from build123d import *

# Parameters (mm, degrees)
BOSS_EXTRUDE1_DEPTH = 1
SKETCH3_R           = 3.15
BOSS_EXTRUDE2_DEPTH = 7.7
FILLET1_R           = 0.3
SKETCH4_W           = 0.65
SKETCH4_H           = 2.8
BOSS_EXTRUDE3_DEPTH = 0.3
BOSS_EXTRUDE4_DEPTH = 0.01


with BuildPart() as part:
    # Sketch2 → Boss-Extrude1 (new body)
    with BuildSketch(Plane(origin=(0, 0, 0), x_dir=(1, 0, 0), z_dir=(0, 1, 0))):
        Polygon((3.3, -3.3), (-3.3, -3.3), (-3.3, 2.25), (-2.25, 3.3), (2.25, 3.3), (3.3, 2.25), align=None)
    extrude(amount=BOSS_EXTRUDE1_DEPTH)

    # Sketch3 → Boss-Extrude2 (add)
    with BuildSketch(Plane(origin=(0, 0, 0), x_dir=(1, 0, 0), z_dir=(0, 1, 0))):
        Circle(SKETCH3_R)
    extrude(amount=BOSS_EXTRUDE2_DEPTH)

    # Fillet1
    fillet1_edges = [part.edges().sort_by_distance(p)[0] for p in [
        (-3.15, 7.7, 0),
    ]]
    fillet(fillet1_edges, radius=FILLET1_R)

    # Sketch4 → Boss-Extrude3 (add)
    with BuildSketch(Plane(origin=(0, 0, 0), x_dir=(1, 0, 0), z_dir=(0, 1, 0))):
        with Locations((0, 2.2)):
            Rectangle(SKETCH4_W, SKETCH4_H)
        with Locations((0, -2.2)):
            Rectangle(SKETCH4_W, SKETCH4_H)
    extrude(amount=BOSS_EXTRUDE3_DEPTH)

    # Sketch5 → Boss-Extrude4 (add)
    with BuildSketch(Plane(origin=(0, 7.7, 0), x_dir=(1, 0, 0), z_dir=(0, 1, 0))):
        with BuildLine():
            Line((-2.494581862, -1.378245745), (2.494581862, -1.378245745))
            ThreePointArc((2.494581862, -1.378245745), (0, -2.85), (-2.494581862, -1.378245745))
        make_face()
    extrude(amount=BOSS_EXTRUDE4_DEPTH)


solid = part.part
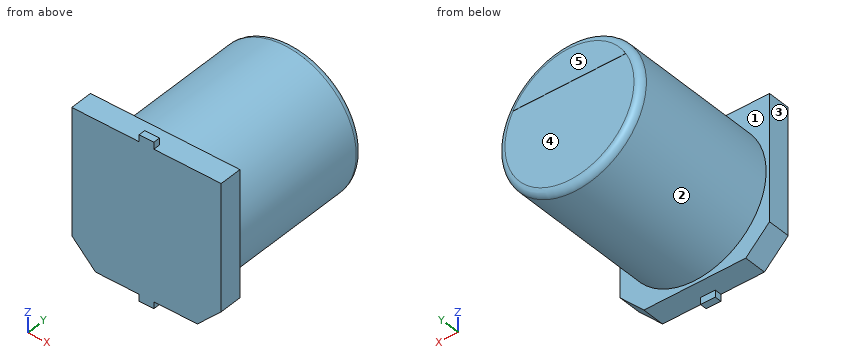
Could you check a few things on this model? Use its own coordinates, in mm. Face numbers are marked on the shaded views. A direction names the side the tool comes from. Round coordinates to 2 decimals unless told otherwise and drop trailing zeros. Write each loop counter-clockwise with the first axis right and the second up, starting at its lowest first coordinate (ties: lowest second). Pieces come first, ordered by that corner, then holes. Notation, with made-up numbers: (20.25, 24) - (33.25, 24) arc R11 ccw to (33.25, 35) - close; hole circle Ø5 at (36, 37.5). An arc over 180 degrees is marked (long way). Put each result on its own line as item: value. Start each with the question number.
(1) I want a section at B-B, the plane y = 0.5. Please give me the cut outline in (x, z), plus the area to 3 significant figures.
(2) I want a section at A-A, the plane z = 0. Please give me the cut outline in (x, y), plus the area to 3 significant figures.
(3) I want a section at D-D, the plane y = 5. Please give me the cut outline in (x, z).
(4) For the marked faces 4 and 5, which set-ups out of +Z, -Z, +X, -X, +Y, -Y let a thin tool reach every point of the face, with its end or its side?
(5) Thinking about a two-plate mould opening in X: for the marked faces 1, 2 and 3, which applies, released by +X, released by -X, zero draft, split by the parting line, or undercut?
(6) I need wall thicknesses on probe 1 along Y at (x, z) = (2, 0); probe 2 along Z at (x, y) = (1, 0.75); probe 3 along Y at (x, z) = (-1.5, -3). Which ranges of each line are inside material? Lowest first, please.
Here are the results:
1. outline: (-3.3, -2.25) - (-2.25, -3.3) - (2.25, -3.3) - (3.3, -2.25) - (3.3, 3.3) - (-3.3, 3.3) - close
1. area: 42.5 mm^2
2. outline: (-3.3, 0) - (3.3, 0) - (3.3, 1) - (3.15, 1) - (3.15, 7.4) arc R0.3 ccw to (2.85, 7.7) - (-2.85, 7.7) arc R0.3 ccw to (-3.15, 7.4) - (-3.15, 1) - (-3.3, 1) - close
2. area: 48.8 mm^2
3. outline: circle Ø6.3 at (0, 0)
4. face 4: -Z, +X, -X, +Y
4. face 5: +Z, -Z, +X, -X, +Y
5. face 1: zero draft
5. face 2: split by the parting line
5. face 3: released by -X
6. probe 1: y = 0 to 7.7
6. probe 2: z = -3.3 to 3.3
6. probe 3: y = 0 to 1
